from build123d import *

# Parameters (mm, degrees)
SKETCH1_W             = 44
SKETCH1_H             = 10
SKETCH1_R             = 1.65
BOSS_EXTRUDE1_DEPTH   = 4
SKETCH2_W             = 44
SKETCH2_H             = 4
BOSS_EXTRUDE2_DEPTH   = 50
RIB6_REACH            = 72.37
SKETCH5_WALL_W        = 158.896391108
SKETCH5_WALL_H        = 3
LPATTERN1_COUNT       = 3
LPATTERN1_PITCH       = 20.5
SKETCH7_W             = 4
SKETCH7_H             = 35
BOSS_EXTRUDE3_DEPTH   = 5
SKETCH8_W             = 4
SKETCH8_H             = 35
BOSS_EXTRUDE4_DEPTH   = 5
FILLET1_R             = 1
SKETCH9_R             = 1.65
CUT_EXTRUDE1_DEPTH    = 74.164198895
LPATTERN2_COUNT       = 4
LPATTERN2_PITCH       = 6
BODY_MOVE_COPY1_ANGLE = 90


with BuildPart() as part:
    # Sketch1 → Boss-Extrude1 (new body)
    with BuildSketch(Plane(origin=(0, 0, 0), x_dir=(1, 0, 0), z_dir=(0, 1, 0))):
        with Locations((22, 5)):
            Rectangle(SKETCH1_W, SKETCH1_H)
        with Locations(Location((38, 3, 0), (0, 0, 270))):
            Circle(SKETCH1_R, mode=Mode.SUBTRACT)
        with Locations(Location((6, 3, 0), (0, 0, 270))):
            Circle(SKETCH1_R, mode=Mode.SUBTRACT)
    extrude(amount=BOSS_EXTRUDE1_DEPTH)

    # Sketch2 → Boss-Extrude2 (add)
    with BuildSketch(Plane(origin=(0, 4, 0), x_dir=(1, 0, 0), z_dir=(0, 1, 0))):
        with Locations((22, 8)):
            Rectangle(SKETCH2_W, SKETCH2_H)
    extrude(amount=BOSS_EXTRUDE2_DEPTH)

    # Sketch5 wall → Rib6 (add, up to next)
    with BuildSketch(Plane(origin=(44, 11.5, -3), x_dir=(0, -0.928476690885, 0.371390676354), z_dir=(0, -0.371390676354, -0.928476690885)), mode=Mode.PRIVATE) as rib6_sk1:
        with Locations((0, 1.5)):
            Rectangle(SKETCH5_WALL_W, SKETCH5_WALL_H)
    rib6_tool1 = extrude(rib6_sk1.sketch, amount=RIB6_REACH, mode=Mode.PRIVATE) - part.part
    rib6 = rib6_tool1.solids().sort_by_distance((44, 11.5, -3))[0]
    add(rib6)

    # LPattern1: Rib6 ×3
    with Locations(*[(-i * LPATTERN1_PITCH, 0, 0) for i in range(1, LPATTERN1_COUNT)]):
        add(rib6)

    # Sketch7 → Boss-Extrude3 (add)
    with BuildSketch(Plane(origin=(44, 0, 0), x_dir=(0, 0, -1), z_dir=(1, 0, 0))):
        with Locations((8, 36.5)):
            Rectangle(SKETCH7_W, SKETCH7_H)
    extrude(amount=BOSS_EXTRUDE3_DEPTH)

    # Sketch8 → Boss-Extrude4 (add)
    with BuildSketch(Plane.ZY):
        with Locations((-8, 36.5)):
            Rectangle(SKETCH8_W, SKETCH8_H)
    extrude(amount=BOSS_EXTRUDE4_DEPTH)

    # Fillet1
    fillet1_edges = [part.edges().sort_by_distance(p)[0] for p in [
        (44, 19, -8),
        (49, 19, -8),
        (49, 54, -8),
        (0, 19, -8),
        (-5, 54, -8),
        (-5, 19, -8),
    ]]
    fillet(fillet1_edges, radius=FILLET1_R)

    # Sketch9 → Cut-Extrude1 (cut, through all)
    with BuildSketch(Plane.XY.offset(-6)):
        with Locations((-0.5, 32)):
            Circle(SKETCH9_R)
        with Locations((44.5, 32)):
            Circle(SKETCH9_R)
    cut_extrude1 = extrude(amount=-CUT_EXTRUDE1_DEPTH, mode=Mode.SUBTRACT)

    # LPattern2: Cut-Extrude1 ×4
    with Locations(*[(0, i * LPATTERN2_PITCH, 0) for i in range(1, LPATTERN2_COUNT)]):
        add(cut_extrude1, mode=Mode.SUBTRACT)


with BuildPart() as part_1:
    # Body-Move/Copy1: moved
    add(part.part.rotate(Axis((0, 27, -5), (1, 0, 0)), BODY_MOVE_COPY1_ANGLE))


solid = part_1.part
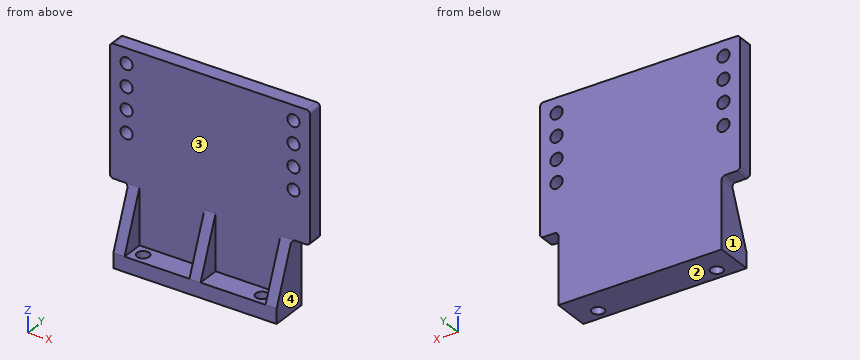
Read the model definition and answer for the solid it produces. Units are mm, in the model's axes. Face numbers are marked on the shaded views. Coordinates: 2 decimals unless noted, no trailing zeros. Loops run counter-clockwise (first coordinate to the right, second up) from the corner with the lowest first, then second, coordinate; pieces in that order, holes last. Notation, with made-up numbers: (52.25, -29) -> (104.25, -29) arc R27 ccw to (104.25, -5) -> close; hole circle Ø11 at (-20.5, -28.75). An arc over 180 degrees is marked (long way). Answer in a Markdown table with one row per item.
Item 1: A cutting plane is placed at C-C on y = 25. Determine the outline of the cut face in (x, z).
Returned:
| item | result |
|---|---|
| outline | (0, -32) -> (4.35, -32) -> (4.35, -28) -> (3, -28) -> (3, -20.5) -> (0, -20.5) -> close; (7.65, -32) -> (36.35, -32) -> (36.35, -28) -> (23.5, -28) -> (23.5, -20.5) -> (20.5, -20.5) -> (20.5, -28) -> (7.65, -28) -> close; (39.65, -32) -> (44, -32) -> (44, -20.5) -> (41, -20.5) -> (41, -28) -> (39.65, -28) -> close |
Item 2: Straight lines are drawn through the part: line 1 along X through (y, z) = (25, -31.05); line 2 along X through (y, z) = (26, -21); line 3 along Z through (x, y) = (-0.5, 30.9). For each, find the intervals that lie inside material, in ascending order. Write a range as [from, to].
Returned:
| item | result |
|---|---|
| line 1 | x = [0, 4.35], [7.65, 36.35], [39.65, 44] |
| line 2 | x = [0, 3], [20.5, 23.5], [41, 44] |
| line 3 | z = [-13.13, -1.65], [1.65, 4.35], [7.65, 10.35], [13.65, 16.35], [19.65, 22] |
Item 3: Each of these flat-tipped pins is pushed along its axis until it touches: P1, Ø1.8, axis at y = 25, z = -19, coming from the +X side; P2, Ø4, axis at x = 38, y = 25, coming from the +Z side; P3, Ø5.5, axis at x = 44.5, z = 0, coming from the -Y side. Where does it stop, or does it pass through?
Returned:
| item | result |
|---|---|
| P1 | stops at x = 44 |
| P2 | stops at z = -28 |
| P3 | stops at y = 28 |
Item 4: For a pull along X with two mould halves and no side action, classify the marked faces 1, 2, 3 and 4 as released by +X, released by -X, zero draft, split by the parting line, or undercut.
Returned:
| item | result |
|---|---|
| face 1 | released by -X |
| face 2 | zero draft |
| face 3 | undercut |
| face 4 | released by +X |
Item 5: A cutting plane is placed at D-D on x = 24.5. Determine the outline of the cut face in (y, z).
Returned:
| item | result |
|---|---|
| outline | (22, -32) -> (32, -32) -> (32, 22) -> (28, 22) -> (28, -28) -> (22, -28) -> close |
Item 6: A cutting plane is placed at A-A on z = 0. Determine the outline of the cut face in (x, y), plus the area to 3 significant figures.
Returned:
| item | result |
|---|---|
| outline | (-5, 28) -> (-2.15, 28) -> (-2.15, 32) -> (-5, 32) -> close; (1.15, 28) -> (42.85, 28) -> (42.85, 32) -> (1.15, 32) -> close; (46.15, 28) -> (49, 28) -> (49, 32) -> (46.15, 32) -> close |
| area | 190 mm^2 |
Item 7: A cutting plane is placed at B-B on x = 6. Determine the outline of the cut face in (y, z).
Returned:
| item | result |
|---|---|
| outline | (22, -32) -> (23.35, -32) -> (23.35, -28) -> (22, -28) -> close; (26.65, -32) -> (32, -32) -> (32, 22) -> (28, 22) -> (28, -28) -> (26.65, -28) -> close |
